Input: dimensioned drawing with shaded views. Units: mm. Origin: part minimum x, y, z. Give positions to 0.01 mm unless a question says otherwise; leave off trailing zeros. Loops run counter-clockwise (first coordinate to the right, second up) from the corner with the lowest first, then second, coordinate; pieces in that order, holes last. Notation, with made-up numbers: M 47.25,78.25 L 56.25,78.25 A24 cw 56.25,99.25 Z; hole C 57,-39 d2. An arc over 180 degrees is marked long. Use CSV: the item, a comma, the result in double quotes. Start each with the question number.
Q1. Section A-A, the plane x = 5. Output: boundary loops of the cut face in (y, z).
Q2. Section D-D, the plane y = 6.25. Output: boundary loops of the cut face in (x, z).
Q3. Pin query (flat end, axial travel): pin 1 (1.5 mm diameter, centred on x = 4, z = 39.5, fed in from -Y); pin 2 (2.5 mm diameter, centred on y = 3.67, z = 44.45, fed in from +X); pin 3 (1.8 mm diameter, centred on y = 3.67, z = 76.2, fed in from +X). Return the tip coordinate at first contact, or that it passes through.
Q4. Section C-C, the plane z = 42.5. Output: boundary loops of the cut face in (x, y).
Q5. Material intervals for line 1 along Y through (x, z) = (4.75, 68); line 2 along Y through (x, z) = (0.65, 44.45) (1 decimal); line 3 along X through (y, z) = (3, 71), sorted ascending.
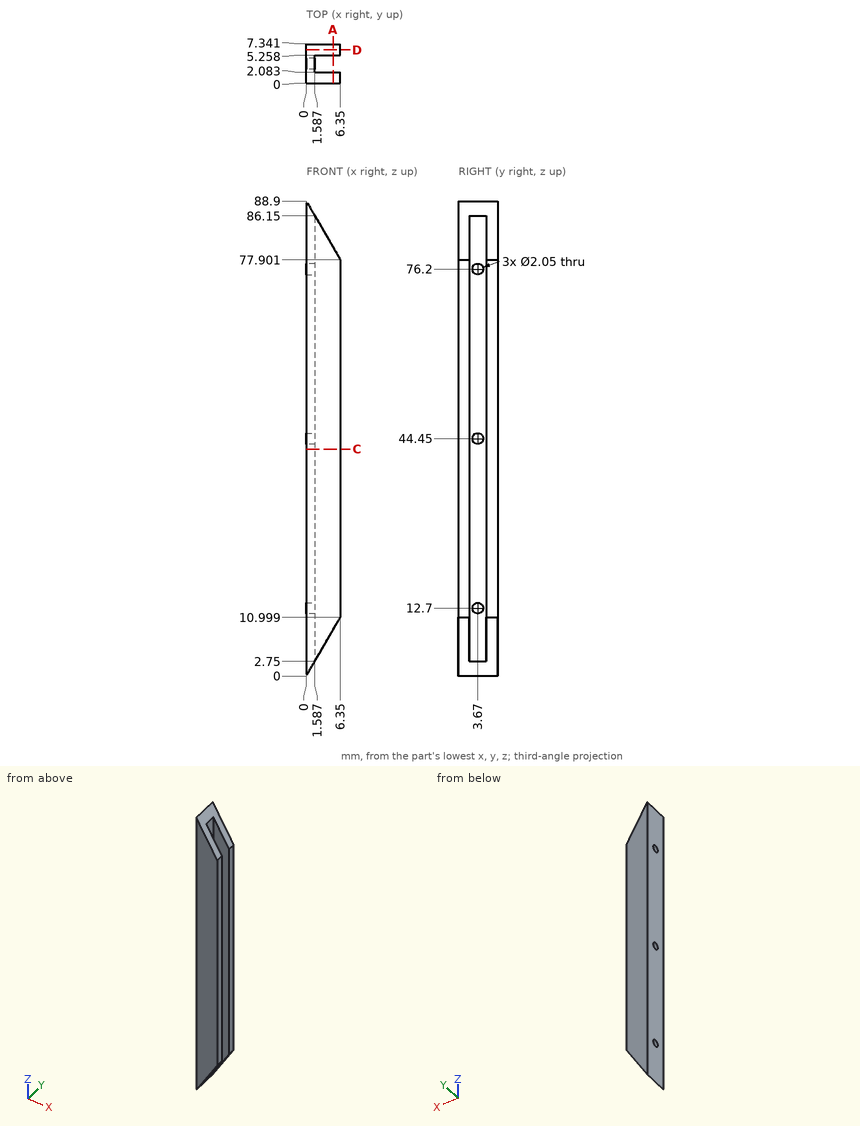
A:
1,outline,"M 0,8.66 L 2.08,8.66 L 2.08,80.24 L 0,80.24 Z; M 5.26,8.66 L 7.34,8.66 L 7.34,80.24 L 5.26,80.24 Z"
2,outline,"M 0,0 L 6.35,11 L 6.35,77.9 L 0,88.9 Z"
3,pin 1,"y = 0"
3,pin 2,"x = 1.59"
3,pin 3,"through"
4,outline,"M 0,0 L 6.35,0 L 6.35,2.08 L 1.59,2.08 L 1.59,5.26 L 6.35,5.26 L 6.35,7.34 L 0,7.34 Z"
5,line 1,"0 to 2.08, 5.26 to 7.34"
5,line 2,"0 to 2.6, 4.7 to 7.3"
5,line 3,"0 to 1.59"
